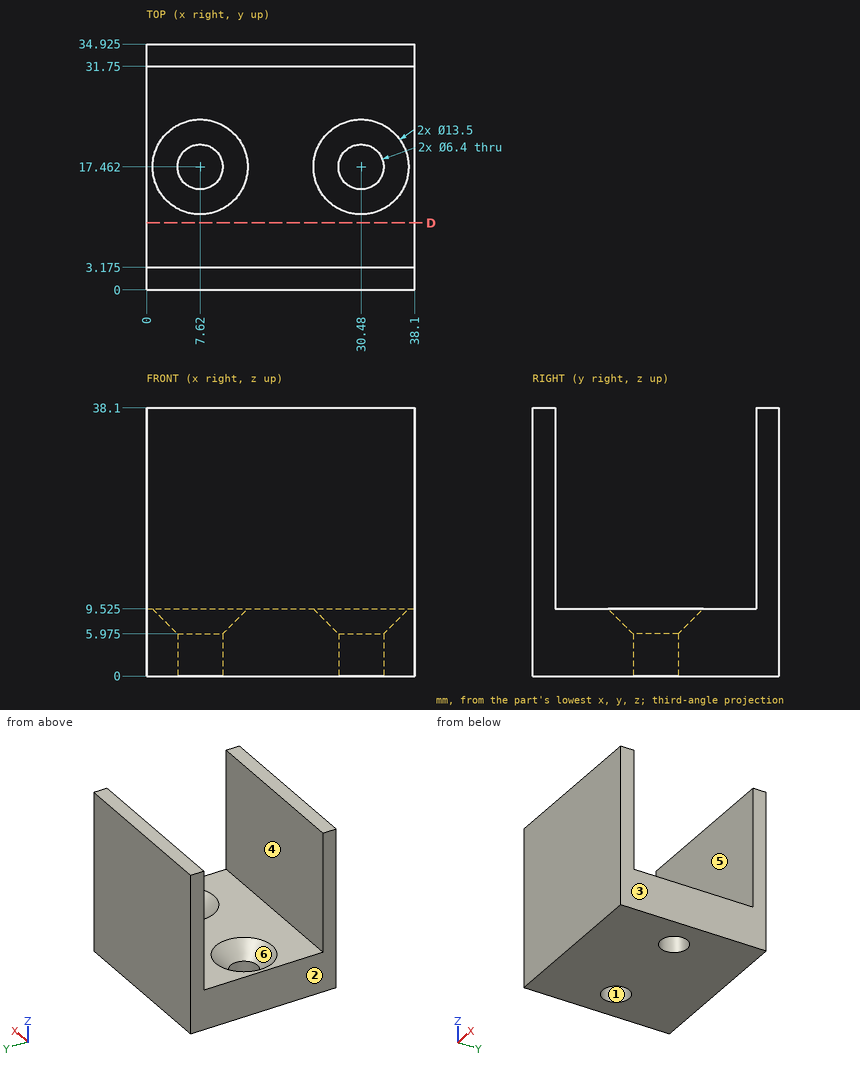
Can you work these out from the drawing? Everything is in mm from the part's minimum corner. A direction names the side the tool comes from. Give positions to 0.01 mm unless a question says otherwise; leave off trailing zeros. Order: outer loops, then holes, each group sorted by start corner. A loop starts at its lowest first (then second) coordinate and runs counter-clockwise, first axis right, second up. Notation, with made-up numbers: M -38.5,11 L -28.5,11 A15 ccw -28.5,27 Z; hole C 65,-2.75 d11. An arc over 180 degrees is marked long. Use a Markdown table: item, result. Add a question column.
Item 1: For the marked faces 5 and 6, which set-ups out of +Z, -Z, +X, -X, +Y, -Y let a thin tool reach every point of the face, with its end or its side?
Item 2: Suppose I cut it at D-D (y = 9.5). List the corners of the cut face in (x, z) for me (1 decimal).
Item 3: Will this pin go through, and if not, where does the flat tip stop? pin 1 (10 mm diameter, centred on y = 18, z = 16.5, fed in from -X).
Item 4: We'd pull the mould along X, two halves only. Please class the marked faces 1, 2, 3 and 4: +X half, -X half, draft (parallel to the pull), parting line (faces both ways), or undercut.
Item 5: If I drill on L1, parallel to Y at x = 7.62, z = 3.65 (1 decimal); L2, parallel to Z at x = 21.5, y = 6 (1 decimal); L3, parallel to Y at x = 7, z = 4 (1 decimal), over which ranges is the centre line in solid material (lowest first)? Write a range as [from, to].
Answer sheet:
| question | item | result |
|---|---|---|
| 1 | face 5 | +Z, +X, -X |
| 1 | face 6 | +Z |
| 2 | outline | M 0,0 L 38.1,0 L 38.1,9.5 L 0,9.5 Z |
| 3 | pin 1 | passes through |
| 4 | face 1 | undercut |
| 4 | face 2 | -X half |
| 4 | face 3 | +X half |
| 4 | face 4 | draft |
| 5 | L1 | y = [0, 14.3], [20.7, 34.9] |
| 5 | L2 | z = [0, 9.5] |
| 5 | L3 | y = [0, 14.3], [20.6, 34.9] |
